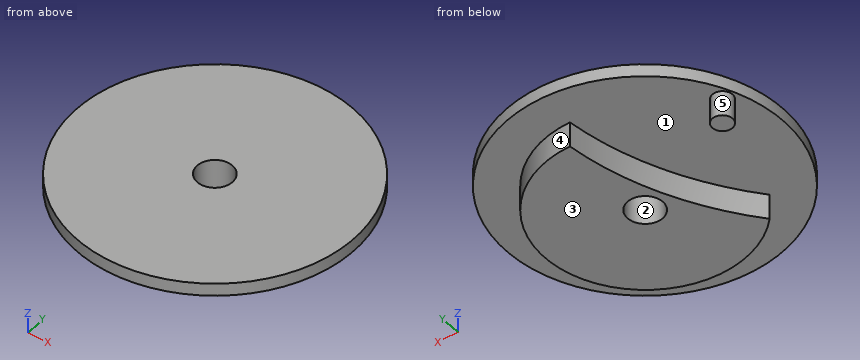
```python
from build123d import *

# Parameters (mm, degrees)
SKETCH1_R             = 4
BOSS_EXTRUDE1_DEPTH   = 10
BOSS_EXTRUDE1_2_DEPTH = 10
SKETCH1_3_R           = 55
BOSS_EXTRUDE2_DEPTH   = 5
SKETCH2_R             = 7
CUT_EXTRUDE1_DEPTH    = 80.277412294


with BuildPart() as part:
    # Sketch1 → Boss-Extrude1 (new body)
    with BuildSketch(Plane.XY):
        with Locations((-46.163581641, 19.207370937)):
            Circle(SKETCH1_R)
    extrude(amount=-BOSS_EXTRUDE1_DEPTH)



with BuildPart() as body_2:
    # Sketch1 → Boss-Extrude1 2 (new body)
    with BuildSketch(Plane.XY):
        with BuildLine():
            ThreePointArc((-28.744125942, -27.906815487), (36.926456917, -15.466500887), (-0.505940955, 39.906800169))
            ThreePointArc((-0.505940955, 39.906800169), (-9.337651898, 3.798280238), (-28.744125942, -27.906815487))
        make_face()
    extrude(amount=-BOSS_EXTRUDE1_2_DEPTH)


with BuildPart() as part_1:
    add(part.part)

    add(body_2.part)  # Boss-Extrude2 merges body 2
    # Sketch1<3> → Boss-Extrude2 (add)
    with BuildSketch(Plane.XY):
        with Locations((0.09, 0)):
            Circle(SKETCH1_3_R)
    extrude(amount=BOSS_EXTRUDE2_DEPTH)

    # Sketch2 → Cut-Extrude1 (cut, through all)
    with BuildSketch(Plane.XY.offset(5)):
        Circle(SKETCH2_R)
    extrude(amount=-CUT_EXTRUDE1_DEPTH, mode=Mode.SUBTRACT)


solid = part_1.part
```
Could you check a few things on this model? Use its own coordinates, in mm. Face numbers are marked on the shaded views. A direction names the side the tool comes from. Round coordinates to 2 decimals unless told otherwise and drop trailing zeros. Order: outer loops, then holes, each group sorted by start corner. A loop starts at its lowest first (then second) coordinate and runs counter-clockwise, first axis right, second up. Notation, with made-up numbers: M 72,78 L 79,78 A28 cw 79,97 Z; hole C 70.25,81 d1. An arc over 180 degrees is marked long. One line per question, with ' | ' between items. Start each with the question number.
(1) For the marked faces 1 and 2, which set-ups out of +Z, -Z, +X, -X, +Y, -Y let a thin tool reach every point of the face, with its end or its side?
(2) Thinking about a two-plate mould opening in X: for the marked faces 3, 4 and 5, which applies, +X half, -X half, draft (parallel to the pull), parting line (faces both ways), or undercut?
(3) Suppose I cut it at B-B on y = 0. List the corners of the cut face in (x, z) for me.
(4) Please list where these lines run through material, in increasing order: line 1 along Y through (x, z) = (0, -1); line 2 along Y through (x, z) = (-0.5, 2.5); line 3 along Z through (x, y) = (-20, 46).
(5) Suppose I cut it at D-D on y = -26.5. List the corners of the cut face in (x, z) for me, then the cut area to 3 significant figures.
(6) Suppose I cut it at C-C on z = 3.25. List the corners of the cut face in (x, y) for me.
(7) For P1, Ø3, axis at x = -25.5, y = 19.5, coming from the -Z side; P2, Ø6, axis at y = 13.5, z = 1.5, coming from the -X side; P3, Ø1, axis at x = -5.5, z = 1.5, coming from the -Y side, each with a flat end and sliding along its axis, tell me the tip position at first contact or that it passes through.
(8) Suppose I cut it at A-A on x = 1.5. List the corners of the cut face in (y, z) for me, then the cut area to 3 significant figures.
Geometry results:
1) face 1: -Z | face 2: +Z, -Z
2) face 3: draft | face 4: parting line | face 5: undercut
3) outline: M -54.91,0 L -11,0 L -11,-10 L -7,-10 L -7,5 L -54.91,5 Z; M 7,-10 L 40,-10 L 40,0 L 55.09,0 L 55.09,5 L 7,5 Z
4) line 1: -40.09 to -7, 7 to 39.91 | line 2: -55 to -6.98, 6.98 to 55 | line 3: 0 to 5
5) outline: M -48.1,0 L -27.57,0 L -27.57,-10 L 30.04,-10 L 30.04,0 L 48.28,0 L 48.28,5 L -48.1,5 Z | area: 1,060 mm²
6) outline: C 0.09,0 d110; hole C 0,0 d14
7) P1: z = 0 | P2: x = -53.9 | P3: y = -54.76
8) outline: M -54.98,0 L -40.06,0 L -40.06,-10 L -6.84,-10 L -6.84,5 L -54.98,5 Z; M 6.84,-10 L 39.88,-10 L 39.88,0 L 54.98,0 L 54.98,5 L 6.84,5 Z | area: 1,140 mm²
